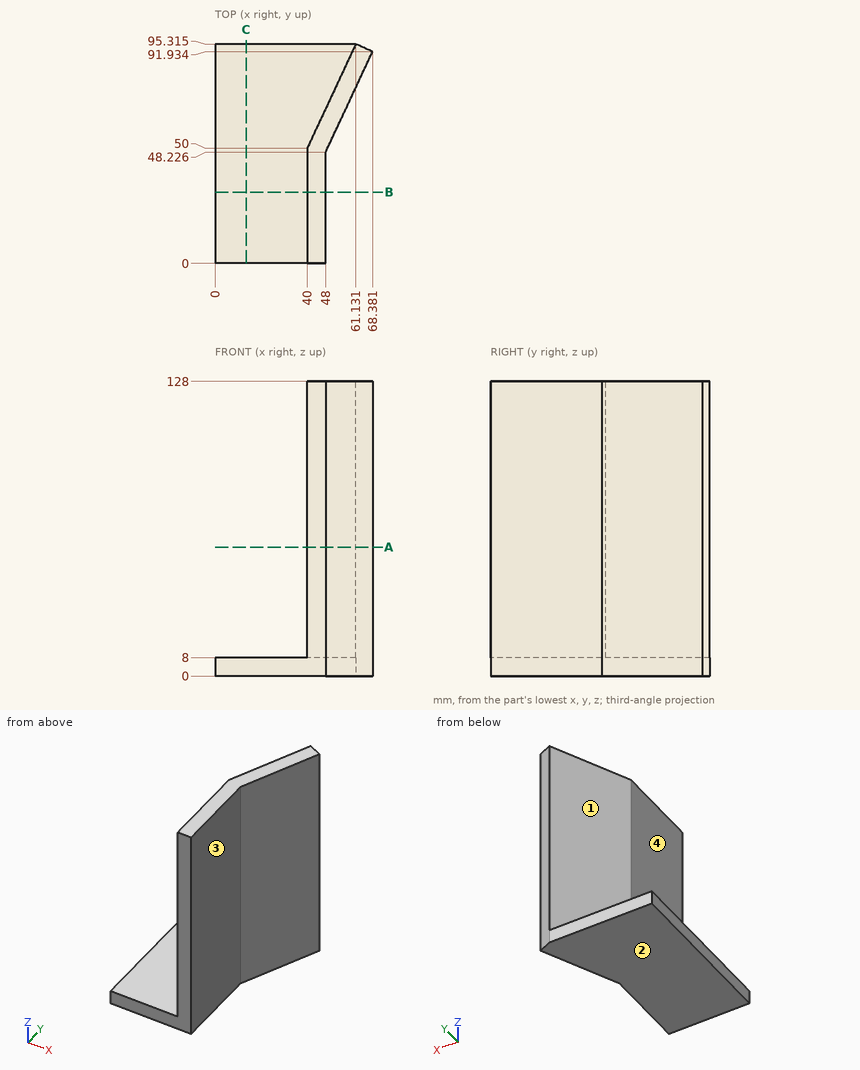
Design review of the part shown in the three views and the two pictorial views. Dimensions are in mm from the part's minimum x, y and z. A direction names the side the tool comes from. Give positions to 0.01 mm unless a question says otherwise; leave off trailing zeros. Loops run counter-clockwise (first coordinate to the right, second up) from the corner with the lowest first, then second, coordinate; pieces in that order, holes last. Notation, with made-up numbers: M 49,-2.75 L 80,-2.75 A25 cw 80,26.25 Z; hole C 43,31.5 d11. An arc over 180 degrees is marked long. Answer as a JSON object with one key per item and string values.
Item 1: Machinability: for the marked faces 1, 2, 3 and 4, which of the approach directions +Z, -Z, +X, -X, +Y, -Y give a long, thin tool a straight path to every point of the face, cutting with its end or side? Answer none if there is none.
Output values:
{"face 1": "+Z, -X, +Y", "face 2": "-Z, +X, -X, +Y, -Y", "face 3": "+Z, -Z, +X, -Y", "face 4": "+Z, -X, +Y, -Y"}
Item 2: We need section B-B (y = 31). State the section outline as (x, z) points.
Output values:
{"outline": "M 0,0 L 48,0 L 48,128 L 40,128 L 40,8 L 0,8 Z"}
Item 3: We need section C-C (x = 13.5). State the section outline as (y, z) points (1 decimal).
Output values:
{"outline": "M 0,0 L 95.3,0 L 95.3,8 L 0,8 Z"}
Item 4: For P1, Ø6, axis at y = 39, z = 84, coming from the -X side; P2, Ø4, axis at x = 59, z = 105, coming from the -Y side (1 decimal); P3, Ø4, axis at y = 26.5, z = 104, coming from the +X side, all flat-tipped, find the tip position at first contact; note any pin that passes through.
Output values:
{"P1": "stops at x = 40", "P2": "stops at y = 67.5", "P3": "stops at x = 48"}
Item 5: We need section A-A (z = 56). State the section outline as (x, y) points (1 decimal).
Output values:
{"outline": "M 40,0 L 48,0 L 48,48.2 L 68.4,91.9 L 61.1,95.3 L 40,50 Z"}
Item 6: Wall thickness on line 1 along Z through (x, y) = (28, 84); line 2 along X through (y, z) = (42.5, 108); line 3 along X through (y, z) = (54, 122) (1 decimal): over which ranges is each line inside the solid? List them lowest first.
Output values:
{"line 1": "z = 0 to 8", "line 2": "x = 40 to 48", "line 3": "x = 41.9 to 50.7"}
